Autodesk Inventor part; units mm, degrees
ref_plane "Work Plane1" through (0, 0, 1.778) normal (0, 0, 1) x (1, 0, 0)
ref_plane "YZ Plane" through (0, 0, 0) normal (1, 0, 0) x (0, 1, 0)
ref_plane "XZ Plane" through (0, 0, 0) normal (0, 1, 0) x (-1, 0, 0)
sketch "Sketch1" plane through (0, 0, 0) normal (0, 0, 1) x (1, 0, 0)
  line L0 (3.048, -1.8479) -> (-3.048, -1.8479)
  line L1 (-3.048, -1.8479) -> (-3.048, 1.8478)
  line L2 (-3.048, 1.8478) -> (3.048, 1.8478)
  line L3 (3.048, 1.8478) -> (3.048, -1.8479)
  line L4 (3.048, -1.8479) -> (-3.048, 1.8478) construction
  line L5 (-3.048, -1.8479) -> (3.048, 1.8478) construction
  point P0 (0, 0)
  dimension "d0" = 6.096
  dimension "d1" = 3.6957
extrude "Extrusion1" add sketch "Sketch1" along normal blind 1.397
sketch "Sketch2" plane through (0, 0, 1.397) normal (0, 0, 1) x (1, 0, 0)
  line L0 (2.286, 1.3653) -> (-2.286, 1.3653)
  line L1 (-2.286, 1.3653) -> (-2.286, -1.3653)
  line L2 (-2.286, -1.3653) -> (2.286, -1.3653)
  line L3 (2.286, -1.3653) -> (2.286, 1.3653)
  line L4 (2.286, 1.3653) -> (-2.286, -1.3653) construction
  line L5 (-2.286, 1.3653) -> (2.286, -1.3653) construction
  point P0 (0, 0)
  dimension "d4" = 4.572
  dimension "d5" = 2.7305
ref_plane "Work Plane1" through (0, 0, 1.778) normal (0, 0, 1) x (1, 0, 0)
sketch "Sketch3" plane through (0, 0, 1.778) normal (0, 0, 1) x (1, 0, 0)
  line L0 (2.0066, 1.143) -> (-2.0066, 1.143)
  line L1 (-2.0066, 1.143) -> (-2.0066, -1.143)
  line L2 (-2.0066, -1.143) -> (2.0066, -1.143)
  line L3 (2.0066, -1.143) -> (2.0066, 1.143)
  line L4 (2.0066, 1.143) -> (-2.0066, -1.143) construction
  line L5 (-2.0066, 1.143) -> (2.0066, -1.143) construction
  point P0 (0, 0)
  dimension "d7" = 4.0132
  dimension "d8" = 2.286
loft "Loft1" add profiles "Sketch2", "Sketch3"
sketch "Sketch4" plane through (-2.0066, 1.143, 1.778) normal (0, 0, 1) x (1, 0, 0)
  line L0 (3.2766, -0.508) -> (0.7366, -0.508)
  line L1 (0.7366, -0.508) -> (0.7366, -1.778)
  line L2 (0.7366, -1.778) -> (3.2766, -1.778)
  line L3 (3.2766, -1.778) -> (3.2766, -0.508)
  line L4 (3.2766, -0.508) -> (0.7366, -1.778) construction
  line L5 (0.7366, -0.508) -> (3.2766, -1.778) construction
  point P0 (2.0066, -1.143)
  dimension "d13" = 2.54
  dimension "d14" = 1.27
extrude "Extrusion2" add sketch "Sketch4" along normal blind 0.635
sketch "Sketch5" plane through (0, 0, 0) normal (0, 1, 0) x (-1, 0, 0)
  line L0 (-3.048, 0) -> (-3.048, 1.397) construction
  line L1 (-3.048, 0.6985) -> (-3.302, 0.6985)
  arc A0 (-3.302, 0.6985) -> (-3.6382, 0.4968) centre (-3.302, 0.3175) ccw
  line L2 (-3.6382, 0.4968) -> (-3.7278, 0.3287)
  arc A1 (-4.064, 0.127) -> (-3.7278, 0.3287) centre (-4.064, 0.508) ccw
  line L3 (3.048, 0) -> (-3.048, 0)
  point P0 (0, 0)
  dimension "d17" = 1.016
  dimension "d18" = 0.127
  dimension "d19" = 0.254
  dimension "d20" = 0.381
sketch "Sketch6" plane through (3.048, -1.8479, 0) normal (1, 0, 0) x (0, 0, -1)
  line L0 (0, 0) -> (-1.397, 0)
  line L1 (-1.397, 0) -> (-1.397, 3.6957)
  line L2 (-0.8255, 2.1019) -> (-0.5715, 2.1019)
  line L3 (-0.5715, 2.1019) -> (-0.5715, 1.5939)
  line L4 (-0.5715, 1.5939) -> (-0.8255, 1.5939)
  line L5 (-0.8255, 1.5939) -> (-0.8255, 2.1019)
  line L6 (-0.8255, 2.1019) -> (-0.5715, 1.5939) construction
  line L7 (-0.5715, 2.1019) -> (-0.8255, 1.5939) construction
  point P0 (0, 1.8479)
  point P1 (-0.6985, 1.8479)
  point P2 (-0.6985, 1.8479)
  point P3 (-0.6985, 1.8479)
  dimension "d21" = 0.254
  dimension "d22" = 0.508
sweep "Sweep1" add profiles "Sketch6" path "Sketch5" path curves L1 A0 L2 A1
mirror "Mirror1" about plane through (0, 0, 0) normal (1, 0, 0) of "Sweep1"
properties part number "Switch"
Read the model definition and answer for the solid it produces. Units are mm, in the model's axes. A direction names the side the tool comes from. Round coordinates to 2 decimals unless told otherwise and drop trailing zeros. Order: outer loops, then holes, each group sorted by start corner. A loop starts at its lowest first (then second) coordinate and runs counter-clockwise, first axis right, second up. Notation, with made-up numbers: (-12, 36.25) - (5, 36.25) arc R22 cw to (5, 55.25) - close; hole circle Ø11 at (29.5, 1.25). An arc over 180 degrees is marked (long way). Use one line per item in the form item = value. Start each with the question number.
(1) For faces 1 (the face through (0, 0, 0)), 2 (the face through (0, -1.6, 1.397)), determine the directions among +Z, -Z, +X, -X, +Y, -Y from which every point of the face is accessible in a straight line to the end or side of a thin tool.
(2) The part is cut by section A-A (x = -2.5). Give the vertices of the cut face in (y, z).
(3) Find the intervals of material crossed by line 1 along Z through (x, y) = (-1.75, -0.8); line 2 along Z through (x, y) = (-2.75, -1.1); line 3 along Y through (x, z) = (-3.5, 0.75), in increasing order. Write a range as from..to.
(4) The part is cut by section B-B (z = 2.2). Give the vertices of the cut face in (x, y) (3 decimals).
(5) Flat-ended cylindrical pins translate along their axes: pin 1 Ø0.7 at (x, z) = (3.5, 0.5) entering from +Y; pin 2 Ø0.7 at (x, z) = (-3.5, 0.5) entering from -Y. Find the tip coordinate at first contact, or state that the pin passes through.
Checked values:
q1.face_1 = -Z, +X, -X, +Y, -Y
q1.face_2 = +Z
q2.outline = (-1.85, 0) - (1.85, 0) - (1.85, 1.4) - (-1.85, 1.4) - close
q3.line_1 = 0..1.78
q3.line_2 = 0..1.4
q3.line_3 = -0.25..0.25
q4.outline = (-1.27, -0.635) - (1.27, -0.635) - (1.27, 0.635) - (-1.27, 0.635) - close
q5.pin_1 = 0.25
q5.pin_2 = -0.25
